```python
from build123d import *

# Parameters (mm, degrees)
SKETCH2_R          = 4
CUT_EXTRUDE1_DEPTH = 20
CHAMFER1_SIZE      = 10
CHAMFER1_SIZE2     = 0.174550649
CHAMFER2_SIZE      = 1


with BuildPart() as part:
    # Sketch1 → Revolve2 (revolve)
    with BuildSketch(Plane(origin=(0, 0, 0), x_dir=(0, 0, -1), z_dir=(1, 0, 0))):
        with BuildLine():
            Line((0, 12), (16, 12))
            ThreePointArc((16, 12), (17.88854382, -8.94427191), (0, -20))
            Line((0, -20), (0, 12))
        make_face()
    revolve(axis=Axis((0, -20, 0), (0, 1, 0)))

    # Sketch2 → Cut-Extrude1 (cut)
    with BuildSketch(Plane(origin=(0, 12, 0), x_dir=(1, 0, 0), z_dir=(0, 1, 0))):
        Circle(SKETCH2_R)
    extrude(amount=-CUT_EXTRUDE1_DEPTH, mode=Mode.SUBTRACT)

    # Chamfer1
    chamfer1_edges = [part.edges().sort_by_distance(p)[0] for p in [
        (-4, -8, 0),
    ]]
    chamfer1_side = [part.faces().sort_by_distance(p)[0] for p in [
        (-4, 2, 0),
    ]]
    chamfer(chamfer1_edges, length=CHAMFER1_SIZE, length2=CHAMFER1_SIZE2, reference=chamfer1_side[0])

    # Chamfer2
    chamfer2_edges = [part.edges().sort_by_distance(p)[0] for p in [
        (-4, 12, 0),
    ]]
    chamfer(chamfer2_edges, length=CHAMFER2_SIZE)


solid = part.part
```
Work out the finished part from the listing and answer in its coordinate system (mm). Coordinates: 2 decimals unless noted, no trailing zeros. Write each loop counter-clockwise with the first axis right and the second up, starting at its lowest first coordinate (ties: lowest second). Pieces come first, ordered by that corner, then holes.
Q1. A cutting plane is placed at B-B, the plane x = 11. Give the vertices of the cut face in (y, z), then the cut area to 3 significant figures.
Q2. A cutting plane is placed at A-A, the plane y = -16. Give the vertices of the cut face in (x, z), then the cut area to 3 significant figures.
Q3. A cutting plane is placed at D-D, the plane y = -0.5. Give the vertices of the cut face in (x, z), then the cut area to 3 significant figures.
Q4. Each of these flat-tipped pins is pushed along its axis until it touches: pin 1 Ø3 at (x, z) = (-11, -13) entering from -Y; pin 2 Ø1 at (y, z) = (-14.5, -10) entering from +X; pin 3 Ø4 at (y, z) = (2, 7) entering from -X; pin 4 Ø4 at (x, z) = (-5, -15.5) entering from +Y. Where does it stop, or does it pass through?
Q5. A cutting plane is placed at C-C, the plane z = 6. Give the vertices of the cut face in (x, y), then the cut area to 3 significant figures.
Q6. Determine the mould class of faces 1 (the face through (0, -8, 0)), 2 (the face through (-4, 12, -4)), 3 (the face through (-0.85, -3.07, 3.82)) for opening direction Z: released by +Z, released by -Z, zero draft, split by the parting line, or undercut.
Q7. Find the intervals of material crossed by line 1 (X direction, y = 6, z = 0); line 2 (X direction, y = 9, z = 0); line 3 (Z direction, x = 0, y = 4), in increasing order.
Findings below:
1. outline: (12, -11.62) - (12, 11.62) arc R16.7 ccw (long way) to start
1. area: 801 mm2
2. outline: circle Ø24 at (0, 0)
2. area: 452 mm2
3. outline: circle Ø39.99 at (0, 0); hole circle Ø7.91 at (0, 0)
3. area: 1,210 mm2
4. pin 1: stops at y = -12.6
4. pin 2: stops at x = 10.35
4. pin 3: stops at x = -19.29
4. pin 4: stops at y = 12
5. outline: (-14.83, 12) arc R19.08 ccw (long way) to (14.83, 12) - close
5. area: 997 mm2
6. face 1: undercut
6. face 2: zero draft
6. face 3: undercut
7. line 1: x = -19.08 to -4, 4 to 19.08
7. line 2: x = -17.86 to -4, 4 to 17.86
7. line 3: z = -19.6 to -4, 4 to 19.6
